For this review, use the dimensioned drawing (mm, ordinates from the lowest corner) and the shaded views. A direction names the side the tool comes from. Round coordinates to 2 decimals unless told otherwise and drop trailing zeros. Loops run counter-clockwise (first coordinate to the right, second up) from the corner with the lowest first, then second, coordinate; pieces in that order, holes last. Notation, with made-up numbers: (53.5, -28) -> (64.5, -28) arc R21 cw to (64.5, 5) -> close; hole circle Ø10 at (-1.75, -14). An arc over 180 degrees is marked (long way). Answer as CSV lines item,"result". Start each with the question number.
(1) Draft analysis for pull direction X (two halves, no side actions). For the marked faces 1, 2 and 3, state which applies: +X half, -X half, draft (parallel to the pull), parting line (faces both ways), or undercut.
(2) Take a section at B-B, the plane z = 15. Write out the cut boundary in (x, y).
(3) Take a section at A-A, the plane y = 19. Write out the cut boundary in (x, z).
(4) For P1, Ø10, axis at y = 12, z = 5, coming from the +X side; P2, Ø1.5, axis at x = 13.5, y = 15, coming from the +Z side; P3, Ø2, axis at x = 16, z = 10.5, coming from the +Y side; P4, Ø1.9, axis at x = 5, y = 19, coming from the +Z side, all flat-tipped, find the tip position at first contact; note any pin that passes through.
(5) To check wall thickness, follow line 1 (X direction, y = 19, z = 0.6); line 2 (Y direction, x = 20, z = 2.55); line 3 (X direction, y = 17.25, z = 3.5). State the ranges of each line that lie inside material, in increasing order. Write a range as from..to.
(6) Take a section at C-C, the plane x = 5. Write out the cut boundary in (y, z), and give its area (3 significant figures).
(7) Machinability: for the marked faces 4, 5 and 6, which of the approach directions +Z, -Z, +X, -X, +Y, -Y give a long, thin tool a straight path to every point of the face, cutting with its end or side? Answer none if there is none.
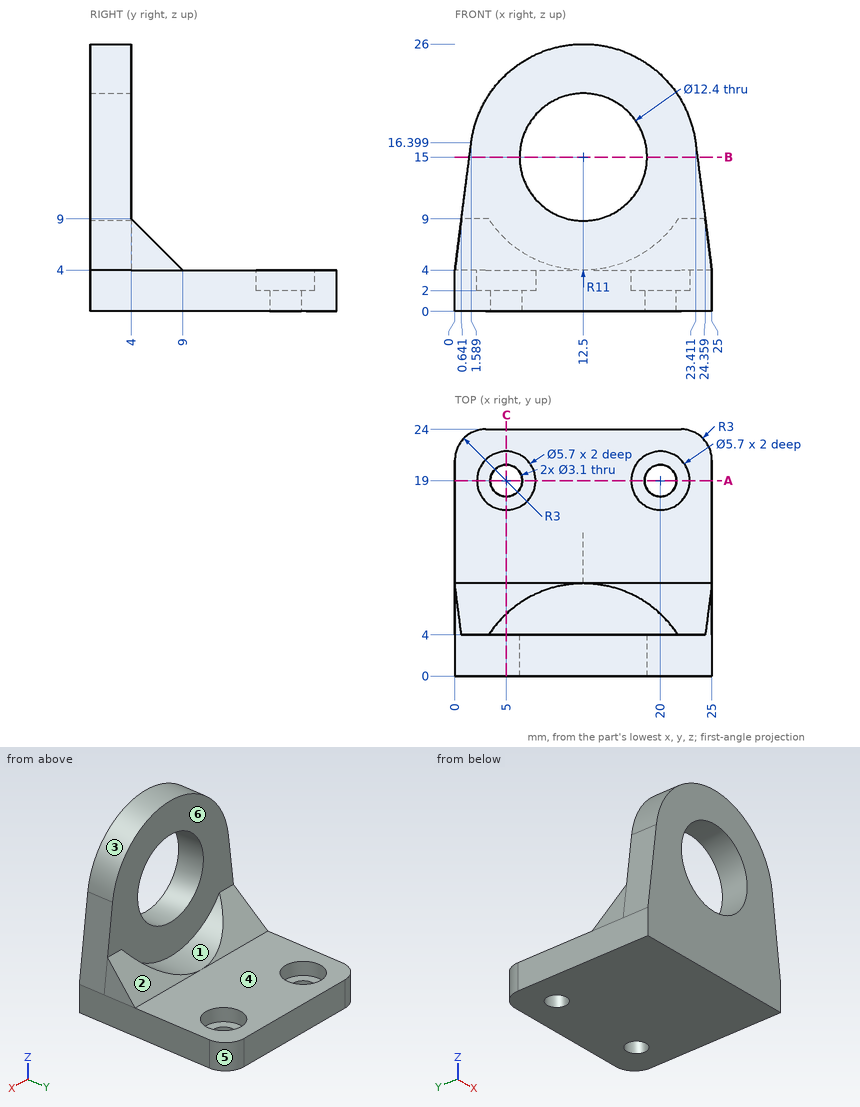
The answers:
1,face 1,"undercut"
1,face 2,"draft"
1,face 3,"parting line"
2,outline,"(1.41, 0) -> (6.3, 0) -> (6.3, 4) -> (1.41, 4) -> close; (18.7, 0) -> (23.59, 0) -> (23.59, 4) -> (18.7, 4) -> close"
3,outline,"(0, 0) -> (3.45, 0) -> (3.45, 2) -> (2.15, 2) -> (2.15, 4) -> (0, 4) -> close; (6.55, 0) -> (18.45, 0) -> (18.45, 2) -> (17.15, 2) -> (17.15, 4) -> (7.85, 4) -> (7.85, 2) -> (6.55, 2) -> close; (21.55, 0) -> (25, 0) -> (25, 4) -> (22.85, 4) -> (22.85, 2) -> (21.55, 2) -> close"
4,P1,"x = 25"
4,P2,"z = 4"
4,P3,"y = 4"
4,P4,"through"
5,line 1,"0..3.45, 6.55..18.45, 21.55..25"
5,line 2,"0..16.15, 21.85..24"
5,line 3,"0..2.75, 7.25..17.75, 22.25..25"
6,outline,"(0, 0) -> (17.45, 0) -> (17.45, 2) -> (16.15, 2) -> (16.15, 4) -> (9, 4) -> (6.05, 6.95) -> (4, 6.95) -> (4, 23.05) -> (0, 23.05) -> close; (20.55, 0) -> (24, 0) -> (24, 4) -> (21.85, 4) -> (21.85, 2) -> (20.55, 2) -> close"
6,area,"165 mm²"
7,face 4,"+Z, +X, -X, +Y"
7,face 5,"+Z, -Z, +X, +Y"
7,face 6,"+Z, +Y"
